Autodesk Inventor part; units mm, degrees
ref_plane "YZ Plane" through (0, 0, 0) normal (1, 0, 0) x (0, 1, 0)
ref_plane "XZ Plane" through (0, 0, 0) normal (0, 1, 0) x (-1, 0, 0)
ref_plane "XY Plane" through (0, 0, 0) normal (0, 0, 1) x (1, 0, 0)
sketch "Sketch1" plane through (0, 0, 0) normal (0, 0, 1) x (1, 0, 0)
  line L0 (-0.0716, 53.5507) -> (107.9284, 53.5507)
  line L1 (107.9284, 53.5507) -> (107.9284, -46.4493)
  line L2 (107.9284, -46.4493) -> (-0.0716, -46.4493)
  line L3 (-0.0716, -46.4493) -> (-0.0716, 53.5507)
  point P0 (0, 0)
  dimension "d0" = 108
  dimension "d1" = 100
extrude "Extrusion1" add sketch "Sketch1" along normal blind 4
sketch "Sketch2" plane through (-0.0716, 53.5507, 0) normal (0, 1, 0) x (1, 0, 0)
  line L0 (0, 0) -> (108, 0)
  line L1 (9.5, 0) -> (28.5, 0)
  line L2 (28.5, 0) -> (28.5, -1.9)
  line L3 (28.5, -1.9) -> (9.5, -1.9)
  line L4 (9.5, -1.9) -> (9.5, 0)
  point P0 (0.0716, 0)
  point P1 (28.5, 0)
  dimension "d4" = 19
  dimension "d5" = 1.9
  dimension "d6" = 9.5
extrude "Extrusion2" add sketch "Sketch2" along normal blind 4
pattern_linear "Rectangular Pattern1" count 3 spacing 35 along (1, 0, 0) count 2 spacing 104 along (0, -1, 0) of "Extrusion2"
sketch "Sketch3" plane through (0, 0, 4) normal (0, 0, 1) x (1, 0, 0)
  line L0 (3.9284, -13.4493) -> (103.9284, -13.4493)
  line L1 (103.9284, -13.4493) -> (103.9284, -34.4493)
  line L2 (103.9284, -34.4493) -> (3.9284, -34.4493)
  line L3 (3.9284, -34.4493) -> (3.9284, -13.4493)
  line L4 (-0.0716, 53.5507) -> (-0.0716, -46.4493)
  line L5 (107.9284, 53.5507) -> (-0.0716, 53.5507)
  line L6 (28.9284, 43.5507) -> (78.9284, 43.5507)
  line L7 (78.9284, 43.5507) -> (78.9284, 33.5507)
  line L8 (78.9284, 33.5507) -> (28.9284, 33.5507)
  line L9 (28.9284, 33.5507) -> (28.9284, 43.5507)
  point P0 (0, 0)
  point P1 (53.9284, -13.4493)
  point P2 (53.9284, 33.5507)
  dimension "d15" = 100
  dimension "d16" = 21
  dimension "d17" = 4
  dimension "d18" = 67
  dimension "d21" = 50
  dimension "d22" = 10
  dimension "d23" = 0
  dimension "d24" = 10
extrude "Extrusion3" cut sketch "Sketch3" against normal blind 4
fillet "Fillet1" radius 5 8 edges at (3.9284, -34.4493, 2) (3.9284, -13.4493, 2) (103.9284, -13.4493, 2) (103.9284, -34.4493, 2) (78.9284, 33.5507, 2) (28.9284, 33.5507, 2) (28.9284, 43.5507, 2) (78.9284, 43.5507, 2)
properties part number "Enclosure_5"
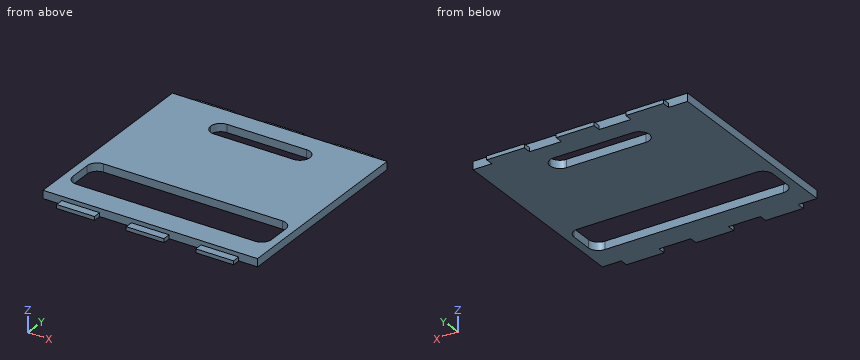
CAD build for the part. Positions are in the model's coordinates, mm. Round coordinates to 2 decimals unless told otherwise and drop trailing zeros. Order: outer loops, then holes, each group sorted by start corner. A loop starts at its lowest first (then second) coordinate and runs counter-clockwise, first axis right, second up. Notation, with made-up numbers: (-5.75, 89.5) - (2.25, 89.5) arc R11 ccw to (2.25, 98.5) - close; hole circle Ø8 at (25, 31.25). An arc over 180 degrees is marked (long way). Use CSV: the item, a comma, the result in double quotes. Start each with the question number.
1) Pin check, flat tips, straight feed: pin 1 Ø2 at (y, z) = (-49.5, 1) entering from -X; pin 2 Ø1.2 at (x, z) = (39.5, 2) entering from -Y; pin 3 Ø1.2 at (x, y) = (53.5, 55) entering from +Z. Stop position of each tip, or through.
2) Wall check: L1, parallel to Y at x = 51, z = 3.2; L2, parallel to X at y = -18.5, z = 1.6; L3, parallel to Y at x = 45, z = 1.1. Give the ranges that are in metal, low to high. Write a range as [from, to].
3) Saw through at C-C (y = -15). List the corners of the cut face in (x, z), and give its area (3 significant figures).
4) Saw through at D-D (z = 3). Count the separate pieces of the cut face and the enclosed holes in it, and give its area (3 significant figures).
5) Saw through at B-B (x = 92). List the corners of the cut face in (y, z), and give its area (3 significant figures).
6) Saw through at A-A (x = 65.5). List the corners of the cut face in (y, z), and give its area (3 significant figures).
Values follow:
1,pin 1,"stops at x = 9.43"
1,pin 2,"stops at y = -46.45"
1,pin 3,"stops at z = 1.9"
2,L1,"y = [-46.45, -34.45], [-13.45, 33.55], [43.55, 53.55]"
2,L2,"x = [-0.07, 3.93], [103.93, 107.93]"
2,L3,"y = [-50.45, -34.45], [-13.45, 33.55], [43.55, 57.55]"
3,outline,"(-0.07, 0) - (5.31, 0) - (5.31, 4) - (-0.07, 4) - close; (102.55, 0) - (107.93, 0) - (107.93, 4) - (102.55, 4) - close"
3,area,"43.0 mm2"
4,separate pieces,"1"
4,enclosed holes,"2"
4,area,"8,240 mm2"
5,outline,"(-50.45, 0) - (-34.45, 0) - (-34.45, 4) - (-46.45, 4) - (-46.45, 1.9) - (-50.45, 1.9) - close; (-13.45, 0) - (57.55, 0) - (57.55, 1.9) - (53.55, 1.9) - (53.55, 4) - (-13.45, 4) - close"
5,area,"331 mm2"
6,outline,"(-46.45, 0) - (-34.45, 0) - (-34.45, 4) - (-46.45, 4) - close; (-13.45, 0) - (33.55, 0) - (33.55, 4) - (-13.45, 4) - close; (43.55, 0) - (53.55, 0) - (53.55, 4) - (43.55, 4) - close"
6,area,"276 mm2"
